Source: CAD feature listing. Evaluate the final solid. Frame: model axes, mm. Face numbers are marked on the shaded views. A direction names the side the tool comes from. Coordinates: 2 decimals unless noted, no trailing zeros. Loops run counter-clockwise (first coordinate to the right, second up) from the corner with the lowest first, then second, coordinate; pieces in that order, holes last. Notation, with made-up numbers: (73.25, 80.5) - (124.25, 80.5) arc R23 cw to (124.25, 88.5) - close; hole circle Ø1 at (24.25, 68.25). An arc over 180 degrees is marked (long way). Write item = value, one per line. Start each with the question number.
from build123d import *

# Parameters (mm, degrees)
F0_W      = 93
F0_H      = 10
F1_DEPTH  = 12
F3_DEPTH  = 90
F5_W      = 8.9714768017
F5_H      = 12
F6_DEPTH  = 1.5
F7_DEPTH  = 2
F8_DEPTH  = 40
F9_W      = 20.4241964966
F9_H      = 12
F10_DEPTH = 4
F11_SIZE  = 3.99999


# Not quite as in the source:
# - a fillet or chamfer is up to 0.001 mm smaller than in the source, because OpenCascade refuses the exact size


with BuildPart() as f1:
    # F0 (on Top) → F1 (new body)
    with BuildSketch(Plane.XY):
        with Locations((46.5, 5)):
            Rectangle(F0_W, F0_H)
    extrude(amount=F1_DEPTH)

    # F2 (on face) → F3 (cut)
    with BuildSketch(Plane.YZ.offset(93)):
        with BuildLine():
            Line((4.8075824627, 6), (4.8075824627, 9.1441176014))
            ThreePointArc((4.8075824627, 9.1441176014), (1.85, 6), (4.8075824627, 2.8558823986))
            Line((4.8075824627, 2.8558823986), (4.8075824627, 6))
        make_face()
        with BuildLine():
            ThreePointArc((5.1924175373, 9.1441176014), (5, 9.15), (4.8075824627, 9.1441176014))
            Line((4.8075824627, 9.1441176014), (5.1924175373, 9.1441176014))
        make_face()
        with BuildLine():
            Line((5.1924175373, 9.1441176014), (4.8075824627, 9.1441176014))
            Line((4.8075824627, 9.1441176014), (4.8075824627, 6))
            Line((4.8075824627, 6), (8.15, 6))
            ThreePointArc((8.15, 6), (7.2944079021, 8.1582845917), (5.1924175373, 9.1441176014))
        make_face()
        with BuildLine():
            Line((5.1924175373, 2.8558823986), (4.8075824627, 2.8558823986))
            ThreePointArc((4.8075824627, 2.8558823986), (5, 2.85), (5.1924175373, 2.8558823986))
        make_face()
        with BuildLine():
            Line((4.8075824627, 6), (4.8075824627, 2.8558823986))
            Line((4.8075824627, 2.8558823986), (5.1924175373, 2.8558823986))
            ThreePointArc((5.1924175373, 2.8558823986), (7.2944079021, 3.8417154083), (8.15, 6))
            Line((8.15, 6), (4.8075824627, 6))
        make_face()
        with BuildLine():
            Line((10, 9.1441176014), (5.1924175373, 9.1441176014))
            ThreePointArc((5.1924175373, 9.1441176014), (7.2944079021, 8.1582845917), (8.15, 6))
            Line((8.15, 6), (10, 6))
            Line((10, 6), (10, 9.1441176014))
        make_face()
        with BuildLine():
            ThreePointArc((8.15, 6), (7.2944079021, 3.8417154083), (5.1924175373, 2.8558823986))
            Line((5.1924175373, 2.8558823986), (10, 2.8558823986))
            Line((10, 2.8558823986), (10, 6))
            Line((10, 6), (8.15, 6))
        make_face()
    extrude(amount=-F3_DEPTH, mode=Mode.SUBTRACT)

    # F5 (on offset) → F6 (cut)
    with BuildSketch(Plane.YZ.offset(33)):
        with Locations((5.5142615992, 6)):
            Rectangle(F5_W, F5_H)
    extrude(amount=F6_DEPTH, mode=Mode.SUBTRACT)

    # F7 (add): a face of the model
    f7_faces = [f1.faces().sort_by_distance(p)[0] for p in [
        (46.5, 0, 6),
    ]]
    extrude(f7_faces, amount=F7_DEPTH)

    # F8 (cut): a face of the model
    f8_faces = [f1.faces().sort_by_distance(p)[0] for p in [
        (93, 4, 0.1697056275),
    ]]
    extrude(f8_faces, amount=-F8_DEPTH, mode=Mode.SUBTRACT)

    # F9 (on face) → F10 (cut)
    with BuildSketch(Plane(origin=(0, 10, 0), x_dir=(-1, 0, 0), z_dir=(0, 1, 0))):
        with Locations((-10.2120982483, 6)):
            Rectangle(F9_W, F9_H)
    extrude(amount=-F10_DEPTH, mode=Mode.SUBTRACT)

    # F11 (size 4 in the source; OpenCascade refuses exactly that, so slightly less here)
    f11_edges = [f1.edges().sort_by_distance(p)[0] for p in [
        (20.424196, 6, 1.427941),
        (20.424196, 6, 10.572059),
    ]]
    chamfer(f11_edges, length=F11_SIZE)


solid = f1.part
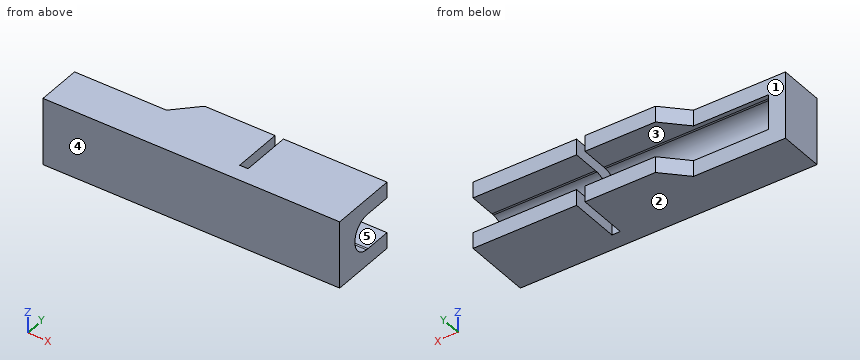
Item 1: Reachability of the marked faces 4 and 5 from +Z, -Z, +X, -X, +Y, -Y: full face, straight path, thin tool, end or side. Return the list, or none.
Item 2: First-contact query: pin 1 (3.5 mm diameter, centred on y = 5, z = 6.5, fed in from +X); pin 2 (1.2 mm diameter, centred on x = 34, z = 7, fed in from +Y). Flat tips, straight axial feed; report the tip coordinate or a pass-through.
Item 3: Cut plane C-C (y = 4). Return the cut outline in (x, z), then the cut area to 3 significant figures.
Item 4: Cut plane D-D (y = 8.5). Return the cut outline in (x, z).
Item 5: Cut plane B-B (z = 6). Return the cut outline in (x, y), then the cut area to 3 significant figures.
Item 6: Material intervals for L1, parallel to Z at x = 8.5, y = 5.5; L2, parallel to X at y = 3.5, z = 9; L3, parallel to X at y = 2.75, z = 7.5, sorted ascending. Write a range as [from, to].
Item 7: Draft query along Z for the marked faces 1, 2 and 3. Return one class per face: released by +Z, released by -Z, zero draft, split by the parting line, or undercut.
Item 8: Cut plane A-A (x = 42.5). Return the cut outline in (y, z).
Responses:
q1.face_4 = +Z, -Z, +X, -X, -Y
q1.face_5 = +X, +Y
q2.pin_1 = 3
q2.pin_2 = 2.15
q3.outline = (0, 0) - (33, 0) - (33, 3.01) - (3, 3.01) - (3, 8.99) - (33, 8.99) - (33, 12) - (0, 12) - close; (34.5, 0) - (53, 0) - (53, 3.01) - (34.5, 3.01) - close; (34.5, 8.99) - (53, 8.99) - (53, 12) - (34.5, 12) - close
q3.area = 328 mm2
q4.outline = (18.92, 0) - (33, 0) - (33, 2.86) - (18.92, 2.86) - close; (18.92, 9.14) - (33, 9.14) - (33, 12) - (18.92, 12) - close; (34.5, 0) - (53, 0) - (53, 2.86) - (34.5, 2.86) - close; (34.5, 9.14) - (53, 9.14) - (53, 12) - (34.5, 12) - close
q5.outline = (0, -2) - (53, -2) - (53, 1.85) - (34.5, 1.85) - (34.5, 1.03) - (33, 1.03) - (33, 1.85) - (3, 1.85) - (3, 6) - (0, 6) - close
q5.area = 215 mm2
q6.L1 = [0, 2.86], [9.14, 12]
q6.L2 = [0, 33], [34.5, 53]
q6.L3 = [0, 3]
q7.face_1 = zero draft
q7.face_2 = released by -Z
q7.face_3 = undercut
q8.outline = (-2, 0) - (10, 0) - (10, 2.86) - (5.19, 2.86) arc R3.15 cw (long way) to (5.19, 9.14) - (10, 9.14) - (10, 12) - (-2, 12) - close
